from build123d import *

# Parameters (mm, degrees)
SKETCH1_R           = 13
BOSS_EXTRUDE1_DEPTH = 65
FILLET1_R           = 1.27
FILLET2_R           = 1.27
SKETCH2_W           = 0.5
SKETCH2_H           = 5
SKETCH2_W_2         = 1
SKETCH2_W_3         = 5
SKETCH2_H_2         = 1
BOSS_EXTRUDE2_DEPTH = 10


with BuildPart() as part:
    # Sketch1 → Boss-Extrude1 (new body)
    with BuildSketch(Plane(origin=(0, 0, 0), x_dir=(1, 0, 0), z_dir=(0, 1, 0))):
        with Locations(Location((0, 0, 0), (0, 0, 270))):
            Circle(SKETCH1_R)
    extrude(amount=BOSS_EXTRUDE1_DEPTH)

    # Fillet1
    fillet1_edges = [part.edges().sort_by_distance(p)[0] for p in [
        (0, 65, -13),
    ]]
    fillet(fillet1_edges, radius=FILLET1_R)

    # Fillet2
    fillet2_edges = [part.edges().sort_by_distance(p)[0] for p in [
        (0, 0, -13),
    ]]
    fillet(fillet2_edges, radius=FILLET2_R)

    # Sketch2 → Boss-Extrude2 (add)
    with BuildSketch(Plane.XY.offset(13)):
        with Locations((-0.25, 5)):
            Rectangle(SKETCH2_W, SKETCH2_H)
        with Locations((0.25, 5)):
            Rectangle(SKETCH2_W, SKETCH2_H)
        with Locations((0, 60)):
            Rectangle(SKETCH2_W_2, SKETCH2_H)
        with Locations((0, 60)):
            Rectangle(SKETCH2_W_3, SKETCH2_H_2)
    extrude(amount=-BOSS_EXTRUDE2_DEPTH)


solid = part.part
The model under review builds one solid part; all positions refer to its coordinate system, in mm. Round coordinates to 2 decimals unless told otherwise and drop trailing zeros. Loops run counter-clockwise (first coordinate to the right, second up) from the corner with the lowest first, then second, coordinate; pieces in that order, holes last. Notation, with made-up numbers: (27, 35) -> (85, 35) arc R32 ccw to (85, 73) -> close; hole circle Ø1 at (86.25, 26.5). An arc over 180 degrees is marked (long way). Return JSON: item names as keys, results as strings.
(1) For pin 1 (6 mm diameter, centred on y = 52.5, z = -6.5, fed in from +X); pin 2 (5 mm diameter, centred on y = 35, z = 3, fed in from +X); pin 3 (2 mm diameter, centred on x = 4.5, y = 36, fed in from +Z), all flat-tipped, find the tip position at first contact; note any pin that passes through.
Solved:
{"pin 1": "x = 12.52", "pin 2": "x = 12.99", "pin 3": "z = 12.52"}
(2) Add section A-A on y = 25. Write out the cut boundary in (x, z).
Solved:
{"outline": "circle Ø26 at (0, 0)"}
(3) For line 1 (Y direction, x = 10, z = 6.5); line 2 (Z direction, x = -1, y = 57); line 3 (X direction, y = 42, z = -6.5), list the stretches that pass through material, from the lowest coordinate up.
Solved:
{"line 1": "0.02 to 64.98", "line 2": "-12.96 to 12.96", "line 3": "-11.26 to 11.26"}
